Part model, mm, in its own coordinate system. A direction names the side the tool comes from. Give positions to 0.01 mm unless a question says otherwise; leave off trailing zeros. Order: outer loops, then holes, each group sorted by start corner. A loop starts at its lowest first (then second) coordinate and runs counter-clockwise, first axis right, second up.
1. Mould opens along X. For faces 1 (the flat face through (7, -4, 5)), 2 (the cylindrical face through (9.139, 14.334, 2.465)), 3 (the conical face through (13.18, -1.29, 2.62)) say: +X half, -X half, draft (parallel to the pull), parting line (faces both ways), or undercut.
2. Slice it at A-A on y = -11.5. List the corners of the cut face in (x, z), and give its area (4 significant figures).
3. Slice it at B-B on x = 0. Give the number of separate pieces and of enclosed holes in the cut face, and give its area (3 significant figures).
4. Which spindle directions (+Z, -Z, +X, -X, +Y, -Y) get a long thin tool onto all of the face, cutting with end or side? Do faces 4 (the cylindrical face through (-7.58, -6.29, 2.47)), 5 (the flat face through (7, 0, 0)). Say none if no direction does.
5. Probe line 1 (Y direction, x = 0, z = 1); line 2 (Y direction, x = 7, z = 2.5); line 3 (X direction, y = 6.5, z = 2). List the from-to ranges inside material, lowest first.
6. Drop flat-ended pins along their axis: pin 1 Ø4 at (x, y) = (-7.78, 7.78) entering from +Z; pin 2 Ø6 at (y, z) = (-8, 55.5) entering from -X; pin 3 Ø6.5 at (x, y) = (11.5, 0) entering from -Z. Give the stop position or say it passes through.
from build123d import *

# Parameters (mm, degrees)
SKETCH1_R                                            = 17
BOSS_EXTRUDE1_DEPTH                                  = 5
SKETCH3_R                                            = 5.2
BOSS_EXTRUDE3_DEPTH                                  = 20
CSK_FOR_M4_HEX_SOCKET_COUNTERSUNK_CAP_SC_D           = 4
CSK_FOR_M4_HEX_SOCKET_COUNTERSUNK_CAP_SC_CSINK_D     = 9
CSK_FOR_M4_HEX_SOCKET_COUNTERSUNK_CAP_SC_CSINK_ANGLE = 90
M4_TAPPED_HOLE1_D                                    = 3
CHAMFER1_SIZE                                        = 0.5
FILLET1_R                                            = 0.3
FILLET2_R                                            = 0.5


with BuildPart() as part:
    # Sketch1 → Boss-Extrude1 (new body)
    with BuildSketch(Plane.XY):
        Circle(SKETCH1_R)
    extrude(amount=BOSS_EXTRUDE1_DEPTH)

    # Sketch3 → Boss-Extrude3 (add)
    with BuildSketch(Plane(origin=(0, 0, 0), x_dir=(-1, 0, 0), z_dir=(0, 0, -1))):
        Circle(SKETCH3_R)
    extrude(amount=BOSS_EXTRUDE3_DEPTH)

    # CSK for M4 Hex Socket Countersunk Cap Screw1 (through all)
    with Locations(Plane.XY.offset(5)):
        with Locations((0, 11.5), (11.5, 0), (0, -11.5), (-11.5, 0)):
            CounterSinkHole(CSK_FOR_M4_HEX_SOCKET_COUNTERSUNK_CAP_SC_D / 2, CSK_FOR_M4_HEX_SOCKET_COUNTERSUNK_CAP_SC_CSINK_D / 2, counter_sink_angle=CSK_FOR_M4_HEX_SOCKET_COUNTERSUNK_CAP_SC_CSINK_ANGLE)

    # M4 Tapped Hole1 (through all)
    with Locations(Plane.XY.offset(5)):
        with Locations((7.778174593, 7.778174593), (-7.778174593, -7.778174593), (-7.778174593, 7.778174593), (7.778174593, -7.778174593)):
            Hole(M4_TAPPED_HOLE1_D / 2)

    # Sketch10 → Revolve1 (revolve)
    with BuildSketch(Plane(origin=(0, 0, 0), x_dir=(0, 0, -1), z_dir=(1, 0, 0))):
        Polygon((-5, 0), (-5, 6), (-61, 6), (-61, 5), (-66, 5), (-66, 4.8), (-67.1, 4.8), (-67.1, 5), (-70, 5), (-70, 0), align=None)
    revolve(axis=Axis((0, 0, -20), (0, 0, 1)))

    # Chamfer1
    chamfer1_edges = [part.edges().sort_by_distance(p)[0] for p in [
        (5.2, 0, -20),
        (0, -5, 70),
    ]]
    chamfer(chamfer1_edges, length=CHAMFER1_SIZE)

    # Fillet1
    fillet1_edges = [part.edges().sort_by_distance(p)[0] for p in [
        (0, -5, 61),
    ]]
    fillet(fillet1_edges, radius=FILLET1_R)

    # Fillet2
    fillet2_edges = [part.edges().sort_by_distance(p)[0] for p in [
        (5.2, 0, 0),
        (0, -6, 5),
    ]]
    fillet(fillet2_edges, radius=FILLET2_R)


solid = part.part
Data:
1. face 1: draft
1. face 2: parting line
1. face 3: undercut
2. outline: (-12.52, 0) - (-2, 0) - (-2, 2.5) - (-4.5, 5) - (-12.52, 5) - close; (2, 0) - (12.52, 0) - (12.52, 5) - (4.5, 5) - (2, 2.5) - close
2. area: 98.95 mm2
3. separate pieces: 3
3. enclosed holes: 0
3. area: 1,090 mm2
4. face 4: +Z, -Z
4. face 5: -Z
5. line 1: y = -17 to -13.5, -9.5 to 9.5, 13.5 to 17
5. line 2: y = -15.49 to -9.06, -6.5 to 6.5, 9.06 to 15.49
5. line 3: x = -15.71 to -8.56, -6.99 to 6.99, 8.56 to 15.71
6. pin 1: stops at z = 5
6. pin 2: stops at x = -3.32
6. pin 3: stops at z = 0
